Autodesk Inventor part; units mm, degrees
ref_plane "YZ Plane" through (0, 0, 0) normal (1, 0, 0) x (0, 1, 0)
ref_plane "XZ Plane" through (0, 0, 0) normal (0, 1, 0) x (-1, 0, 0)
ref_plane "XY Plane" through (0, 0, 0) normal (0, 0, 1) x (1, 0, 0)
sketch "スケッチ1" plane through (0, 0, 0) normal (0, 0, 1) x (1, 0, 0)
  line L0 (0, 3.1754) -> (2.75, 1.5877)
  line L1 (2.75, 1.5877) -> (2.75, -1.5877)
  line L2 (2.75, -1.5877) -> (0, -3.1754)
  line L3 (0, -3.1754) -> (-2.75, -1.5877)
  line L4 (-2.75, -1.5877) -> (-2.75, 1.5877)
  line L5 (-2.75, 1.5877) -> (0, 3.1754)
  point P0 (0, 0)
  point P1 (0, 0)
  dimension "d0" = 5.5
extrude "押し出し1" add sketch "スケッチ1" along normal blind 80
sketch "スケッチ2" plane through (0, 0, 80) normal (0, 0, 1) x (1, 0, 0)
  point P0 (0, 0)
hole "穴1" at (0, 0, 80) direction (0, 0, -1) diameter 2.459 depth 8.8 tip angle 118
sketch "スケッチ3" plane through (0, 0, 0) normal (0, 0, -1) x (-1, 0, 0)
  point P0 (0, 0)
hole "穴2" at (0, 0, 0) direction (0, 0, 1) diameter 2.459 depth 8.8 tip angle 118
properties part number "アルミスペーサー(六角・酸洗処理）_ASL-380E" material "アルミニウム 6061"
Part model, mm, in its own coordinate system. A direction names the side the tool comes from. Coordinates: 2 decimals unless noted, no trailing zeros. Order: outer loops, then holes, each group sorted by start corner. A loop starts at its lowest first (then second) coordinate and runs counter-clockwise, first axis right, second up. Notation, with made-up numbers: M 28,25 L 40,25 A29 cw 40,55 Z; hole C 33,7.25 d11. An arc over 180 degrees is marked long. Use a Markdown table: item, result.
(1) Flat gauge pins, fed straight in: pin 1 (2 mm diameter, centred on x = 2, z = 66, fed in from +Y); pin 2 (1.5 mm diameter, centred on x = -0.5, z = 27.5, fed in from -Y); pin 3 (1.5 mm diameter, centred on x = 0, y = 0, fed in from +Z). Where does each tip first touch, or does it go through?
A:
| item | result |
|---|---|
| pin 1 | stops at y = 2.6 |
| pin 2 | stops at y = -3.18 |
| pin 3 | stops at z = 70.91 |
(2) Pull direction Y, two halves, no side cores. Call faces 1 (the flat face through (0, -1.4, 80)), 2 (the cylindrical face through (0.748, 0.976, 75.538)), 3 (the flat face through (1.36, 2.39, 39.44)): released by +Y, released by -Y, zero draft, split by the parting line, or undercut.
A:
| item | result |
|---|---|
| face 1 | zero draft |
| face 2 | undercut |
| face 3 | released by +Y |
(3) Cut at B-B on z = 61.5. Write the cut outline in (x, y), then the cut area to 3 significant figures.
A:
| item | result |
|---|---|
| outline | M -2.75,-1.59 L 0,-3.18 L 2.75,-1.59 L 2.75,1.59 L 0,3.18 L -2.75,1.59 Z |
| area | 26.2 mm^2 |
(4) Cut at C-C on y = 2.5. Write the cut outline in (x, z), then the cut area to 3 significant figures.
A:
| item | result |
|---|---|
| outline | M -1.17,0 L 1.17,0 L 1.17,80 L -1.17,80 Z |
| area | 187 mm^2 |
(5) Probe L1, parallel to X at y = 0, z = 2.5; L2, parallel to Y at x = 0, z = 5.5; L3, parallel to X at y = 2.25, z = 8. List the from-to ranges inside material, lowest first.
A:
| item | result |
|---|---|
| L1 | x = -2.75 to -1.23, 1.23 to 2.75 |
| L2 | y = -3.18 to -1.23, 1.23 to 3.18 |
| L3 | x = -1.6 to 1.6 |
(6) Cut at A-A on z = 72. Write the cut outline in (x, y), then the cut area to 3 significant figures.
A:
| item | result |
|---|---|
| outline | M -2.75,-1.59 L 0,-3.18 L 2.75,-1.59 L 2.75,1.59 L 0,3.18 L -2.75,1.59 Z; hole C 0,0 d2.46 |
| area | 21.4 mm^2 |
(7) Tool access for faces 4 (the cylindrical face through (0.748, -0.976, 4.462)), 5 (the flat face through (2.75, 0, 39)): list every direction of +Z, -Z, +X, -X, +Y, -Y with a clear straight run to the whole face (end or side of a thin tool).
A:
| item | result |
|---|---|
| face 4 | -Z |
| face 5 | +Z, -Z, +X, +Y, -Y |
